from build123d import *

# Parameters (mm, degrees)
F1_DEPTH = 63.5
F2_DEPTH = 25.4
F3_DEPTH = 15.875
F5_R     = 6.35


with BuildPart() as f1:
    # F0 (on Front) → F1 (new body, symmetric)
    with BuildSketch(Plane.XZ):
        Polygon((22.225, 9.525), (-41.275, 9.525), (-41.275, -9.525), (41.275, -9.525), (41.275, 9.525), align=None)
    extrude(amount=F1_DEPTH, both=True)

    # F0 (on Front) → F2 (join, symmetric)
    with BuildSketch(Plane.XZ):
        with BuildLine():
            Line((22.225, 30.275552), (22.225, 9.525))
            Line((22.225, 9.525), (41.275, 9.525))
            Line((41.275, 9.525), (41.275, 30.275552))
            ThreePointArc((41.275, 30.275552), (45.421853, 39.644869), (55.145303, 42.8752))
            Line((55.145303, 42.8752), (60.325, 42.8752))
            Line((60.325, 42.8752), (60.325, 61.9252))
            Line((60.325, 61.9252), (55.853148, 61.9252))
            add(Edge.make_bspline(
                [(50.991166, 61.84665), (52.640021, 61.916743), (54.262423, 61.943544), (55.853148, 61.9252)],
                knots=[105.839839, 105.839839, 105.839839, 105.839839, 110.361488, 110.361488, 110.361488, 110.361488], degree=3))
            ThreePointArc((50.991166, 61.84665), (30.495036, 51.631035), (22.225, 30.275552))
        make_face()
        Polygon((85.725, 61.9252), (60.325, 61.9252), (60.325, 42.8752), (82.916974, 42.8752), (85.725, 42.8752), align=None)
    extrude(amount=F2_DEPTH, both=True)

    # F0 (on Front) → F3 (join)
    with BuildSketch(Plane.XZ):
        with BuildLine():
            add(Edge.make_bspline(
                [(-41.275, 9.525), (-40.69288, 34.845239), (12.395848, 60.205958), (50.991166, 61.84665)],
                knots=[0, 0, 0, 0, 105.839839, 105.839839, 105.839839, 105.839839], degree=3))
            Line((-41.275, 9.525), (22.225, 9.525))
            Line((22.225, 9.525), (22.225, 30.275552))
            ThreePointArc((22.225, 30.275552), (30.495036, 51.631035), (50.991166, 61.84665))
        make_face()
    extrude(amount=F3_DEPTH)

    # F0 (on Front) → F4 (revolve)
    with BuildSketch(Plane.XZ):
        Polygon((85.725, 66.675), (85.725, 61.9252), (85.725, 42.8752), (85.725, 38.1), (111.125, 38.1), (111.125, 66.675), align=None)
    revolve(axis=Axis((85.725, 0, 52.3875), (0, 0, 1)))

    # F5
    f5_edges = [f1.edges().sort_by_distance(p)[0] for p in [
        (41.275, -63.5, 0),
        (41.275, 63.5, 0),
        (-41.275, -63.5, 0),
        (-41.275, 63.5, 0),
    ]]
    fillet(f5_edges, radius=F5_R)


solid = f1.part
Geometry check sheet. Reference: the model listing, model coordinates, mm. A direction names the side the tool comes from. Round coordinates to 2 decimals unless told otherwise and drop trailing zeros. Write each loop counter-clockwise with the first axis right and the second up, starting at its lowest first coordinate (ties: lowest second). Pieces come first, ordered by that corner, then holes.
Item 1: Go/stop test with flat-tipped pins: pin 1 Ø10 at (y, z) = (42, 7.5) entering from +X (3 decimals); pin 2 Ø7.5 at (y, z) = (-20, 19.5) entering from -X (3 decimals); pin 3 Ø1 at (x, y) = (53, -13) entering from -Z. Record where each tip stops, or that it passes through.
Determined:
pin 1: stops at x = 41.275
pin 2: stops at x = 22.225
pin 3: stops at z = 42.85
Item 2: Section check A-A (y = -53). Record the boundary of the cut face in (x, z) (3 decimals), plus the area to 3 significant figures.
Determined:
outline: (-41.275, -9.525) - (41.275, -9.525) - (41.275, 9.525) - (-41.275, 9.525) - close
area: 1,570 mm2
Item 3: Mould release check, pull along X, two halves, no side actions. Record for faces 1 (the face through (1, -40, 9.525)), 2 (the face through (60, -2, 42.875)), 3 (the face through (30.717, 12.522, 51.872)): +X half, -X half, draft (parallel to the pull), parting line (faces both ways), or undercut.
Determined:
face 1: draft
face 2: undercut
face 3: -X half
Item 4: Access from +Z, -Z, +X, -X, +Y, -Y to the whole of each face (thin tool, end or side, straight path). Record for faces 4 (the face through (46, 25.4, 42)), 5 (the face through (30.717, -20.704, 51.872)), 6 (the face through (86, 0, 38.1)).
Determined:
face 4: +Z, +X, -X, +Y
face 5: +Z, -X, -Y
face 6: -Z, +X, +Y, -Y
Item 5: Material ranges on line 1 along X through (y, z) = (-25.5, 8) (3 decimals); line 2 along Z through (x, y) = (-27, 5) (3 decimals); line 3 along Z through (x, y) = (90, 4) (3 decimals), recorded low to high.
Determined:
line 1: x = -41.275 to 41.275
line 2: z = -9.525 to 9.525
line 3: z = 38.1 to 66.675
